Source: CAD feature listing. Evaluate the final solid. Frame: model axes, mm. A direction names the side the tool comes from. Coordinates: 2 decimals unless noted, no trailing zeros. Order: outer loops, then holes, each group sorted by start corner. A loop starts at its lowest first (then second) coordinate and runs counter-clockwise, first axis right, second up.
```python
from build123d import *

# Parameters (mm, degrees)
SKETCH1_W               = 45
SKETCH1_H               = 20
BRACKETBASE_DEPTH       = 5
SKETCH3_R               = 1.375
MOUNTINGTABS_DEPTH      = 5
SKETCH4_W               = 15
SKETCH4_H               = 5
HEADERSLOT_DEPTH        = 13.625
SKETCH6_R               = 2.5
CUT_EXTRUDE1_DEPTH      = 3.25
CUT_EXTRUDE1_DEPTH_BACK = 21


with BuildPart() as part:
    # Sketch1 → bracketBase (new body)
    with BuildSketch(Plane(origin=(0, 0, 0), x_dir=(1, 0, 0), z_dir=(0, 1, 0))):
        with Locations((22.5, 10)):
            Rectangle(SKETCH1_W, SKETCH1_H)
    extrude(amount=BRACKETBASE_DEPTH)

    # Sketch2 → ballPoint1 (revolve)
    with BuildSketch(Plane(origin=(0, 5, 0), x_dir=(1, 0, 0), z_dir=(0, 1, 0))):
        with BuildLine():
            Line((12.25, 13.25), (12.25, 6.75))
            ThreePointArc((12.25, 6.75), (9, 10), (12.25, 13.25))
        make_face()
    ballpoint1 = revolve(axis=Axis((12.25, 5, -13.25), (0, 0, 1)))

    # Mirror1: ballPoint1 across plane
    add(ballpoint1.mirror(Plane.ZY.offset(-22.5)))

    # Sketch3 → mountingTabs (add)
    with BuildSketch(Plane.XZ):
        Polygon((45, -20), (53.5, -11.75), (53.5, 2.25), (47.5, 2.25), (47.5, 0), (45, 0), align=None)
        with Locations((50.5, -0.75)):
            Circle(SKETCH3_R, mode=Mode.SUBTRACT)
        with Locations((50.5, -7.75)):
            Circle(SKETCH3_R, mode=Mode.SUBTRACT)
        Polygon((-2.5, 0), (0, 0), (0, -20), (-8.5, -11.75), (-8.5, 2.25), (-2.5, 2.25), align=None)
        with Locations((-5.5, -0.75)):
            Circle(SKETCH3_R, mode=Mode.SUBTRACT)
        with Locations((-5.5, -7.75)):
            Circle(SKETCH3_R, mode=Mode.SUBTRACT)
    extrude(amount=-MOUNTINGTABS_DEPTH)

    # Sketch4 → headerSlot (cut)
    with BuildSketch(Plane.XZ):
        with Locations((22.5, -17.5)):
            Rectangle(SKETCH4_W, SKETCH4_H)
    extrude(amount=-HEADERSLOT_DEPTH, mode=Mode.SUBTRACT)

    # Sketch6 → Cut-Extrude1 (cut, two sides)
    with BuildSketch(Plane.XY) as cut_extrude1_sk:
        with Locations((44.5, 0)):
            Circle(SKETCH6_R)
        with Locations((0.5, 0)):
            Circle(SKETCH6_R)
    extrude(amount=CUT_EXTRUDE1_DEPTH, mode=Mode.SUBTRACT)
    extrude(cut_extrude1_sk.sketch, amount=-CUT_EXTRUDE1_DEPTH_BACK, mode=Mode.SUBTRACT)


solid = part.part
```
1. Section query D-D on y = 7.5. Return loops of the section in (x, z).
Findings:
outline: circle Ø4.15 at (12.25, -10); circle Ø4.15 at (32.75, -10)
2. Ray query, line 1 (Z direction, x = 50.5, y = 3.9) (3 decimals); line 2 (X direction, y = 4, z = -1); line 3 (X direction, y = 3.75, z = -1.5). Return the intervals inside material, ascending.
Findings:
line 1: z = -14.662 to -9.125, -6.375 to -2.125, 0.625 to 2.25
line 2: x = -8.5 to -6.85, -4.15 to 49.15, 51.85 to 53.5
line 3: x = -8.5 to -6.65, -4.35 to 49.35, 51.65 to 53.5
3. Pin query (flat end, axial travel): P1, Ø6, axis at x = 21.5, z = -10, coming from the +Y side; P2, Ø4, axis at x = -1, z = 0, coming from the -Y side; P3, Ø2, axis at x = 50.5, z = -7.75, coming from the -Y side; P4, Ø1.5, axis at y = 3, z = -17.5, coming from the -X side. Return the tip coordinate at first contact, or that it passes through.
Findings:
P1: stops at y = 5
P2: stops at y = 0
P3: passes through
P4: stops at x = -3.35
4. Section query A-A on z = -0.75. Return loops of the section in (x, y) (3 decimals), plus the area to 3 significant figures.
Findings:
outline: (-8.5, 0) - (-6.875, 0) - (-6.875, 5) - (-8.5, 5) - close; (-4.125, 0) - (-2, 0) arc R2.5 cw to (3, 0) - (42, 0) arc R2.5 cw to (47, 0) - (49.125, 0) - (49.125, 5) - (-4.125, 5) - close; (51.875, 0) - (53.5, 0) - (53.5, 5) - (51.875, 5) - close
area: 263 mm2
5. Access query for faces 1 (the face through (23, 2, 0)), 2 (the face through (49.19, 2.465, -15.933)), 3 (the face through (30, 2, -18)). Directions: +Z, -Z, +X, -X, +Y, -Y. A direction counts if a zero-diameter tool reaches every point of the face in a straight line with its end or side. Return the directions, or none.
Findings:
face 1: +Z, +Y, -Y
face 2: -Z, +X, +Y, -Y
face 3: -Z, +Y, -Y
6. Section query C-C on x = 50.5. Return loops of the section in (y, z) (3 decimals), plus the area to 3 significant figures.
Findings:
outline: (0, -14.662) - (5, -14.662) - (5, -9.125) - (0, -9.125) - close; (0, -6.375) - (5, -6.375) - (5, -2.125) - (0, -2.125) - close; (0, 0.625) - (5, 0.625) - (5, 2.25) - (0, 2.25) - close
area: 57.1 mm2
7. Draft query along Z for faces 4 (the face through (0.6, 2.5, -9.9)), 5 (the face through (22, 2, -15)), 6 (the face through (49.126, 2.465, -7.69)). Return one class per face: released by +Z, released by -Z, zero draft, split by the parting line, or undercut.
Findings:
face 4: zero draft
face 5: released by -Z
face 6: undercut
8. Section query B-B on y = 1.5. Return loops of the section in (x, z) (3 decimals).
Findings:
outline: (-8.5, -11.75) - (-1.5, -18.544) - (-1.5, 0) - (-2.5, 0) - (-2.5, 2.25) - (-8.5, 2.25) - close; (2.5, -20) - (15, -20) - (15, -15) - (30, -15) - (30, -20) - (42.5, -20) - (42.5, 0) - (2.5, 0) - close; (46.5, -18.544) - (53.5, -11.75) - (53.5, 2.25) - (47.5, 2.25) - (47.5, 0) - (46.5, 0) - close; hole circle Ø2.75 at (-5.5, -7.75); hole circle Ø2.75 at (-5.5, -0.75); hole circle Ø2.75 at (50.5, -7.75); hole circle Ø2.75 at (50.5, -0.75)
